Design review of the part shown in the three views and the two pictorial views. Dimensions are in mm from the part's minimum x, y and z. A direction names the side the tool comes from. Give positions to 0.01 mm unless a question says otherwise; leave off trailing zeros. Loops run counter-clockwise (first coordinate to the right, second up) from the corner with the lowest first, then second, coordinate; pieces in that order, holes last.
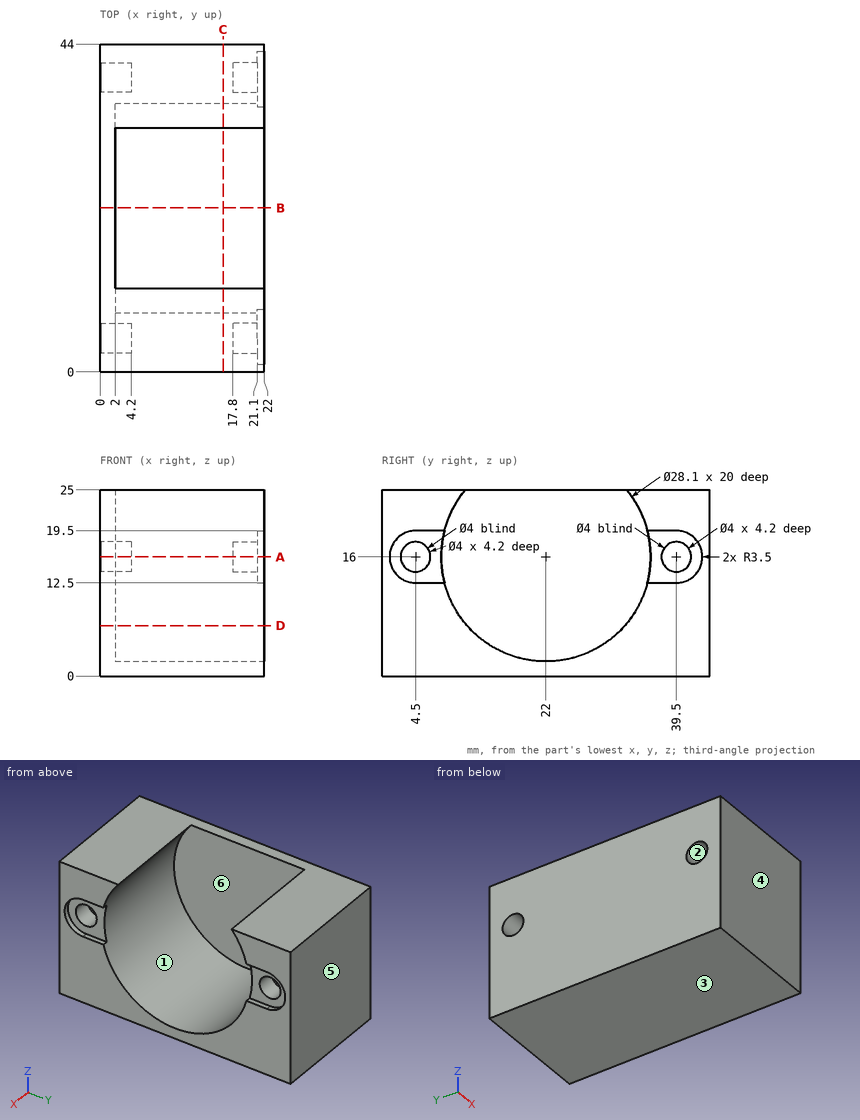
Q1. Wall thickness on line 1 (Y direction, x = 3.5, z = 19.5); line 2 (Z direction, x = 1.25, y = 4.5); line 3 (X direction, y = 8, z = 17.5): over which ranges is each line inside the solid? List them lowest first.
Results:
line 1: y = 0 to 8.39, 35.61 to 44
line 2: z = 0 to 14, 18 to 25
line 3: x = 0 to 21.1
Q2. Take a section at D-D (z = 6.75). Give the boundary of the cut face in (x, y), plus the area to 3 significant figures.
Results:
outline: (0, 0) - (22, 0) - (22, 11.42) - (2, 11.42) - (2, 32.58) - (22, 32.58) - (22, 44) - (0, 44) - close
area: 545 mm2
Q3. Tool access review of the marked faces 1, 2 and 3: name each direction out of +Z, -Z, +X, -X, +Y, -Y from which nothing blocks a thin tool from reaching the whole face with its end or side.
Results:
face 1: +X
face 2: -X
face 3: -Z, +X, -X, +Y, -Y
Q4. Insertion check: pin 1 (2 mm diameter, centred on y = 26, z = 18, fed in from +X); pin 2 (1.5 mm diameter, centred on x = 13.5, z = 9.5, fed in from -Y); pin 3 (3.5 mm diameter, centred on y = 5.5, z = 17, fed in from +X); pin 4 (2 mm diameter, centred on y = 39, z = 15.5, fed in from -X). Each pin has a flat end and moves straight along its axis. Give the tip position at first contact, or say it passes through.
Results:
pin 1: stops at x = 2
pin 2: stops at y = 0
pin 3: stops at x = 21.1
pin 4: stops at x = 4.2
Q5. Take a section at A-A (z = 16). Give the boundary of the cut face in (x, y).
Results:
outline: (0, 0) - (22, 0) - (22, 1) - (21.1, 1) - (21.1, 2.5) - (17.8, 2.5) - (17.8, 6.5) - (21.1, 6.5) - (21.1, 7.95) - (2, 7.95) - (2, 36.05) - (21.1, 36.05) - (21.1, 37.5) - (17.8, 37.5) - (17.8, 41.5) - (21.1, 41.5) - (21.1, 43) - (22, 43) - (22, 44) - (0, 44) - (0, 41.5) - (4.2, 41.5) - (4.2, 37.5) - (0, 37.5) - (0, 6.5) - (4.2, 6.5) - (4.2, 2.5) - (0, 2.5) - close
Q6. Take a section at B-B (y = 22). Give the boundary of the cut face in (x, z), plus the area to 3 significant figures.
Results:
outline: (0, 0) - (22, 0) - (22, 1.95) - (2, 1.95) - (2, 25) - (0, 25) - close
area: 89.0 mm2
Q7. Take a section at C-C (x = 16.5). Give the boundary of the cut face in (y, z).
Results:
outline: (0, 0) - (44, 0) - (44, 25) - (32.79, 25) arc R14.05 cw (long way) to (11.21, 25) - (0, 25) - close
Q8. Draft analysis for pull direction Y (two halves, no side actions). For the marked faces 4, 5 and 6, state which applies: pulls with the +Y half, pulls with the -Y half, needs draft (parallel to the pull), parting line crosses it, or undercut.
Results:
face 4: pulls with the -Y half
face 5: pulls with the +Y half
face 6: undercut
